Model file for the job. Use its own axes, mm. A direction names the side the tool comes from. Coordinates: 2 decimals unless noted, no trailing zeros. Write each loop counter-clockwise with the first axis right and the second up, starting at its lowest first coordinate (ties: lowest second). Pieces come first, ordered by that corner, then holes. Notation, with made-up numbers: M -24,10 L 24,10 A22 ccw 24,23 Z; hole C 27.5,89.25 d7. An arc over 180 degrees is marked long. One line per question, with ' | ' between items. Start each with the question number.
(1) Tool access for faces 1 (the face through (-35.683, 1.838, 27.857)), 2 (the face through (-93.849, 9.268, 54.053)), 3 (the face through (-85.8, 9.514, 27.857)): list every direction of +Z, -Z, +X, -X, +Y, -Y with a clear straight run to the whole face (end or side of a thin tool).
(2) Wall check: probe 1 along Z at (x, y) = (-163, 39); probe 2 along Y at (x, z) = (-166, 47.5); probe 3 along X at (y, z) = (-30, 6.5). Give the ranges that are in metal, low to high.
(3) Cut at A-A (z = 37.5). Count the separate pieces of the cut face and the enclosed holes in it, plus the area to 3 significant figures.
(4) Cut at B-B (y = -37). Write the cut outline in (x, z), plus the area to 3 significant figures.
(5) Cut at C-C (x = -15.5). Write the cut outline in (y, z).
(6) Flat gauge pins, fed straight in: pin 1 Ø1 at (y, z) = (-15, 13) entering from +X; pin 2 Ø16.5 at (y, z) = (-28, 18) entering from -X; pin 3 Ø12 at (x, z) = (-180.5, 24.5) entering from +Y. Where does each tip first touch, or does it go through?
(7) Two-plate mould, pull along X, no slides. Class faces 4 (the face through (-22.755, 0.319, 27.857)), 5 (the face through (-86, -115.623, 28)), 6 (the face through (-170.674, 45.454, 53.986)): +X half, -X half, draft (parallel to the pull), parting line (faces both ways), or undercut.
from build123d import *

# Parameters (mm, degrees)
BOSS_EXTRUDE1_DEPTH = 55
SKETCH2_W           = 51
SKETCH2_H           = 56
CUT_EXTRUDE1_DEPTH  = 198.600505619
BOSS_EXTRUDE4_DEPTH = 55
SKETCH7_W           = 239.563416731
SKETCH7_H           = 55
BOSS_EXTRUDE5_DEPTH = 10
CHAMFER6_SIZE       = 2
CHAMFER7_SIZE       = 2
FILLET4_R           = 5
FILLET5_R           = 5
FILLET6_R           = 5
FILLET7_R           = 5


# Some blends are built 0.0001 mm under size
with BuildPart() as part:
    # Sketch1 → Boss-Extrude1 (new body)
    with BuildSketch(Plane.XY):
        Polygon((0, 0), (-174.334072166, 15.252254981), (-169.104727601, 75.023936866), (5.229344565, 59.771681886), align=None)
    extrude(amount=BOSS_EXTRUDE1_DEPTH)

    # Sketch2 → Cut-Extrude1 (cut, through all)
    with BuildSketch(Plane(origin=(0, 0, 0), x_dir=(0, 0, -1), z_dir=(0.9961946980917452, -0.08715574274766201, 0))):
        with Locations((-27.5, 30)):
            Rectangle(SKETCH2_W, SKETCH2_H)
    extrude(amount=-CUT_EXTRUDE1_DEPTH, mode=Mode.SUBTRACT)

    # Sketch3 → Boss-Extrude4 (add)
    with BuildSketch(Plane.XY):
        Polygon((-164.334072166, 14.377368346), (-164.334072166, -105.622631654), (-154.334072166, -105.622631654), (-154.334072166, 13.50248171), align=None)
        Polygon((-34.334072166, 3.003842087), (-34.334072166, -105.622631654), (-24.334072166, -105.622631654), (-24.334072166, 2.128955452), align=None)
    extrude(amount=BOSS_EXTRUDE4_DEPTH)

    # Sketch7 → Boss-Extrude5 (add)
    with BuildSketch(Plane.XZ.offset(105.622631654)):
        with Locations((-84.5523638, 27.5)):
            Rectangle(SKETCH7_W, SKETCH7_H)
    extrude(amount=BOSS_EXTRUDE5_DEPTH)

    # Chamfer6
    chamfer6_edges = [part.edges().sort_by_distance(p)[0] for p in [
        (-169.279039087, 73.03154747, 27.5),
        (-171.719399884, 45.138095924, 53),
        (-174.159760681, 17.244644377, 27.5),
        (-171.719399884, 45.138095924, 2),
        (2.614672282, 29.885840943, 2),
        (5.055033079, 57.779292489, 27.5),
        (2.614672282, 29.885840943, 53),
        (0.174311485, 1.992389396, 27.5),
    ]]
    chamfer(chamfer6_edges, length=CHAMFER6_SIZE - 0.0001)  # a hair under: the kernel refuses the full size

    # Chamfer7
    # the kernel refuses this chamfer: 2 mm, written as the material it takes off along each edge
    with BuildSketch(Plane(origin=(-159.21027825, 13.929094464, 55), x_dir=(-0.0023964235484937708, -0.027391246498851614, -0.9996219169112968), z_dir=(-0.9961946980917452, 0.08715574274766169, 0))) as chamfer7_piece_1_section:
        Polygon((CHAMFER7_SIZE * 0.999621916911, -CHAMFER7_SIZE * 0.0274958766106), (-CHAMFER7_SIZE * 0.0274958766106, -CHAMFER7_SIZE * 0.999621916911), (0, 0), align=None)
    chamfer7_piece_1 = extrude(amount=20.324930327, mode=Mode.PRIVATE)
    chamfer7_piece_1 = split(chamfer7_piece_1, bisect_by=Plane(origin=(-164.334072166, 15.69707124, 54.339627198), z_dir=(-1, 0, 0)), keep=Keep.TOP, mode=Mode.PRIVATE)
    add(chamfer7_piece_1, mode=Mode.SUBTRACT)
    with BuildSketch(Plane(origin=(-29.21027825, 2.555568205, 0), x_dir=(0.08712279063524543, 0.9958180537233409, -0.02749587661058642), z_dir=(-0.9961946980917452, 0.08715574274766169, 0))) as chamfer7_piece_2_section:
        Polygon((CHAMFER7_SIZE * 0.999621916911, -CHAMFER7_SIZE * 0.0274958766106), (-CHAMFER7_SIZE * 0.0274958766106, -CHAMFER7_SIZE * 0.999621916911), (0, 0), align=None)
    chamfer7_piece_2 = extrude(amount=130.745112457, mode=Mode.PRIVATE)
    chamfer7_piece_2 = split(chamfer7_piece_2, bisect_by=Plane(origin=(-34.334072166, 8.915268669, 0.659587254), z_dir=(-1, 0, 0)), keep=Keep.TOP, mode=Mode.PRIVATE)
    chamfer7_piece_2 = split(chamfer7_piece_2, bisect_by=Plane(origin=(-154.334072166, 8.915268669, 0.659587254), z_dir=(1, 0, 0)), keep=Keep.TOP, mode=Mode.PRIVATE)
    add(chamfer7_piece_2, mode=Mode.SUBTRACT)
    with BuildSketch(Plane(origin=(5.123793916, -0.448273882, 0), x_dir=(0.08712279063524543, 0.9958180537233409, -0.027495876610586438), z_dir=(-0.9961946980917452, 0.08715574274766169, 0))) as chamfer7_piece_3_section:
        Polygon((CHAMFER7_SIZE * 0.999621916911, -CHAMFER7_SIZE * 0.0274958766106), (-CHAMFER7_SIZE * 0.0274958766106, -CHAMFER7_SIZE * 0.999621916911), (0, 0), align=None)
    chamfer7_piece_3 = extrude(amount=34.71375632, mode=Mode.PRIVATE)
    chamfer7_piece_3 = split(chamfer7_piece_3, bisect_by=Plane(origin=(-24.334072166, 1.500682903, 0.659186265), z_dir=(1, 0, 0)), keep=Keep.TOP, mode=Mode.PRIVATE)
    add(chamfer7_piece_3, mode=Mode.SUBTRACT)
    with BuildSketch(Plane(origin=(-29.21027825, 2.555568205, 55), x_dir=(0.08712279063524543, 0.9958180537233409, 0.02749587661058574), z_dir=(-0.9961946980917452, 0.08715574274766169, 0))) as chamfer7_piece_4_section:
        Polygon((CHAMFER7_SIZE * 0.999621916911, CHAMFER7_SIZE * 0.0274958766106), (-CHAMFER7_SIZE * 0.0274958766106, CHAMFER7_SIZE * 0.999621916911), (0, 0), align=None)
    chamfer7_piece_4 = extrude(amount=130.745112457, mode=Mode.PRIVATE)
    chamfer7_piece_4 = split(chamfer7_piece_4, bisect_by=Plane(origin=(-34.334072166, 8.915268669, 54.340412746), z_dir=(-1, 0, 0)), keep=Keep.TOP, mode=Mode.PRIVATE)
    chamfer7_piece_4 = split(chamfer7_piece_4, bisect_by=Plane(origin=(-154.334072166, 8.915268669, 54.340412746), z_dir=(1, 0, 0)), keep=Keep.TOP, mode=Mode.PRIVATE)
    add(chamfer7_piece_4, mode=Mode.SUBTRACT)
    with BuildSketch(Plane(origin=(5.123793916, -0.448273882, 55), x_dir=(0.08712279063524543, 0.9958180537233409, 0.02749587661058574), z_dir=(-0.9961946980917452, 0.08715574274766169, 0))) as chamfer7_piece_5_section:
        Polygon((CHAMFER7_SIZE * 0.999621916911, CHAMFER7_SIZE * 0.0274958766106), (-CHAMFER7_SIZE * 0.0274958766106, CHAMFER7_SIZE * 0.999621916911), (0, 0), align=None)
    chamfer7_piece_5 = extrude(amount=34.71375632, mode=Mode.PRIVATE)
    chamfer7_piece_5 = split(chamfer7_piece_5, bisect_by=Plane(origin=(-24.334072166, 1.500682903, 54.340813735), z_dir=(1, 0, 0)), keep=Keep.TOP, mode=Mode.PRIVATE)
    add(chamfer7_piece_5, mode=Mode.SUBTRACT)
    with BuildSketch(Plane(origin=(-159.21027825, 13.929094464, 0), x_dir=(-0.002396423548493694, -0.02739124649885074, 0.9996219169112968), z_dir=(-0.9961946980917452, 0.08715574274766169, 0))) as chamfer7_piece_6_section:
        Polygon((CHAMFER7_SIZE * 0.999621916911, CHAMFER7_SIZE * 0.0274958766106), (-CHAMFER7_SIZE * 0.0274958766106, CHAMFER7_SIZE * 0.999621916911), (0, 0), align=None)
    chamfer7_piece_6 = extrude(amount=20.324930327, mode=Mode.PRIVATE)
    chamfer7_piece_6 = split(chamfer7_piece_6, bisect_by=Plane(origin=(-164.334072166, 15.69707124, 0.660372802), z_dir=(-1, 0, 0)), keep=Keep.TOP, mode=Mode.PRIVATE)
    add(chamfer7_piece_6, mode=Mode.SUBTRACT)
    with BuildSketch(Plane(origin=(-174.228521517, 75.472210748, 0), x_dir=(-0.08712279063524556, -0.9958180537233409, -0.02749587661058637), z_dir=(0.9961946980917452, -0.08715574274766183, 0))) as chamfer7_piece_7:
        Polygon((CHAMFER7_SIZE * 0.999621916911, -CHAMFER7_SIZE * 0.0274958766106), (-CHAMFER7_SIZE * 0.0274958766106, -CHAMFER7_SIZE * 0.999621916911), (0, 0), align=None)
    extrude(amount=185.286731952, mode=Mode.SUBTRACT)
    with BuildSketch(Plane(origin=(-174.228521517, 75.472210748, 55), x_dir=(-0.08712279063524556, -0.9958180537233409, 0.02749587661058563), z_dir=(0.9961946980917452, -0.08715574274766183, 0))) as chamfer7_piece_8:
        Polygon((CHAMFER7_SIZE * 0.999621916911, CHAMFER7_SIZE * 0.0274958766106), (-CHAMFER7_SIZE * 0.0274958766106, CHAMFER7_SIZE * 0.999621916911), (0, 0), align=None)
    extrude(amount=185.286731952, mode=Mode.SUBTRACT)

    # Fillet4
    fillet4_edges = [part.edges().sort_by_distance(p)[0] for p in [
        (-24.334072166, 2.128955452, 27.5),
    ]]
    fillet(fillet4_edges, radius=FILLET4_R)

    # Fillet5
    fillet5_edges = [part.edges().sort_by_distance(p)[0] for p in [
        (-34.334072166, 3.003842087, 27.5),
    ]]
    fillet(fillet5_edges, radius=FILLET5_R)

    # Fillet6
    fillet6_edges = [part.edges().sort_by_distance(p)[0] for p in [
        (-154.334072166, 13.50248171, 27.5),
    ]]
    fillet(fillet6_edges, radius=FILLET6_R)

    # Fillet7
    fillet7_edges = [part.edges().sort_by_distance(p)[0] for p in [
        (-164.334072166, 14.377368346, 27.5),
    ]]
    fillet(fillet7_edges, radius=FILLET7_R)


solid = part.part
Filled in:
1) face 1: +Z, -Z | face 2: +Z | face 3: +X
2) probe 1: 0 to 2, 53 to 55 | probe 2: -115.62 to -105.62, 13.52 to 16.53, 72.74 to 74.75 | probe 3: -164.33 to -154.33, -34.33 to -24.33
3) separate pieces: 2 | enclosed holes: 1 | area: 5,390 mm²
4) outline: M -164.33,0 L -154.33,0 L -154.33,55 L -164.33,55 Z; M -34.33,0 L -24.33,0 L -24.33,55 L -34.33,55 Z | area: 1,100 mm²
5) outline: M -115.62,0 L -105.62,0 L -105.62,55 L -115.62,55 Z; M 1.36,2 L 3.36,0 L 59.58,0 L 61.59,2 L 61.59,53 L 59.58,55 L 3.36,55 L 1.36,53 Z; hole M 3.36,2 L 59.58,2 L 59.58,53 L 3.36,53 Z
6) pin 1: x = -24.33 | pin 2: x = -164.33 | pin 3: y = -105.62
7) face 4: undercut | face 5: draft | face 6: -X half
